from build123d import *

# Parameters (mm, degrees)
F0_W     = 762
F0_H     = 647.7
F1_DEPTH = 314.325
F2_R     = 22.225
F3_DEPTH = 114.3
F4_W     = 762
F4_H     = 12.7
F5_DEPTH = 114.3
F6_W     = 762
F6_H     = 647.7
F6_W_2   = 755.65
F6_H_2   = 641.35
F7_DEPTH = 15.875


with BuildPart() as f1:
    # F0 (on Front) → F1 (new body, symmetric)
    with BuildSketch(Plane.XZ):
        with Locations((0, 438.15)):
            Rectangle(F0_W, F0_H)
    extrude(amount=F1_DEPTH, both=True)

    # F2 (on Top) → F3 (join)
    with BuildSketch(Plane.XY):
        with Locations((-304.8, -238.125)):
            Circle(F2_R)
        with Locations((304.8, -238.125)):
            Circle(F2_R)
        with Locations((304.8, 238.125)):
            Circle(F2_R)
        with Locations((-304.8, 238.125)):
            Circle(F2_R)
    extrude(amount=F3_DEPTH)

    # F4 (on Top) → F5 (join, through all)
    with BuildSketch(Plane.XY):
        with Locations((0, -266.954)):
            Rectangle(F4_W, F4_H)
    extrude(amount=F5_DEPTH)

    # F6 (on face) → F7 (cut)
    with BuildSketch(Plane.XZ.offset(314.325)):
        with Locations((0, 438.15)):
            Rectangle(F6_W, F6_H)
        with Locations((0, 438.15)):
            Rectangle(F6_W_2, F6_H_2, mode=Mode.SUBTRACT)
    extrude(amount=-F7_DEPTH, mode=Mode.SUBTRACT)


solid = f1.part
Input: part model. Units: mm. Frame: model coordinates. A direction names the side the tool comes from. Give positions to 0.01 mm unless a question says otherwise; leave off trailing zeros. Loops run counter-clockwise (first coordinate to the right, second up) from the corner with the lowest first, then second, coordinate; pieces in that order, holes last. Notation, with made-up numbers: (15.5, -8.75) -> (45.5, -8.75) arc R21 cw to (45.5, 21.25) -> close; hole circle Ø5 at (4.25, 23). An arc over 180 degrees is marked (long way). Answer as a JSON object with one key per item and string values. Group by question number.
Item 1: Pull-direction query (X, two-part tool) for faces 4 (the cylindrical face through (-294.54, 218.41, 56.35)), 5 (the flat face through (304, 238, 0)), 6 (the flat face through (381, 4, 376)); classes: released by +X, released by -X, zero draft, split by the parting line, or undercut.
Item 2: Line query: probe 1 along Y at (x, z) = (124.5, 77.5); probe 2 along Z at (x, y) = (-216, 57). Output: solid intervals per line, ascending.
Item 3: Cut plane B-B, the plane y = -168.5. Return the cut outline in (x, z), and give its area (3 significant figures).
Item 4: Pin query (flat end, axial travel): P1, Ø10, axis at x = 113.5, y = -9, coming from the -Z side; P2, Ø17.5, axis at y = -309.5, z = 563, coming from the +X side (3 decimals); P3, Ø17.5, axis at x = 158.5, y = -309, coming from the +Z side (3 decimals). Return the tip coordinate at first contact, or that it passes through.
Item 5: Reachability of faces 1 (the cylindrical face through (287.163, 224.601, 56.35)), 2 (the flat face through (-5, -314.325, 443)), 3 (the flat face through (-5, -273.304, 56)) from +Z, -Z, +X, -X, +Y, -Y: full face, straight path, thin tool, end or side. Return the list, or none.
Item 6: Cut plane C-C, the plane x = -304.8. Return the cut outline in (y, z) (3 decimals).
Item 7: Cut plane A-A, the plane x = -198.5. Return the cut outline in (y, z) (3 decimals).
Checks:
{
 "1": {"face 4": "undercut", "face 5": "zero draft", "face 6": "released by +X"},
 "2": {"probe 1": "y = -273.3 to -260.6", "probe 2": "z = 114.3 to 762"},
 "3": {"outline": "(-381, 114.3) -> (381, 114.3) -> (381, 762) -> (-381, 762) -> close", "area": "494,000 mm²"},
 "4": {"P1": "stops at z = 114.3", "P2": "stops at x = 377.825", "P3": "stops at z = 758.825"},
 "5": {"face 1": "-Z", "face 2": "+Z, -Z, +X, -X, -Y", "face 3": "-Z, +X, -X, -Y"},
 "6": {"outline": "(-314.325, 117.475) -> (-298.45, 117.475) -> (-298.45, 114.3) -> (-273.304, 114.3) -> (-273.304, 0) -> (-260.604, 0) -> (-260.604, 114.3) -> (-260.35, 114.3) -> (-260.35, 0) -> (-215.9, 0) -> (-215.9, 114.3) -> (215.9, 114.3) -> (215.9, 0) -> (260.35, 0) -> (260.35, 114.3) -> (314.325, 114.3) -> (314.325, 762) -> (-298.45, 762) -> (-298.45, 758.825) -> (-314.325, 758.825) -> close"},
 "7": {"outline": "(-314.325, 117.475) -> (-298.45, 117.475) -> (-298.45, 114.3) -> (-273.304, 114.3) -> (-273.304, 0) -> (-260.604, 0) -> (-260.604, 114.3) -> (314.325, 114.3) -> (314.325, 762) -> (-298.45, 762) -> (-298.45, 758.825) -> (-314.325, 758.825) -> close"}
}
